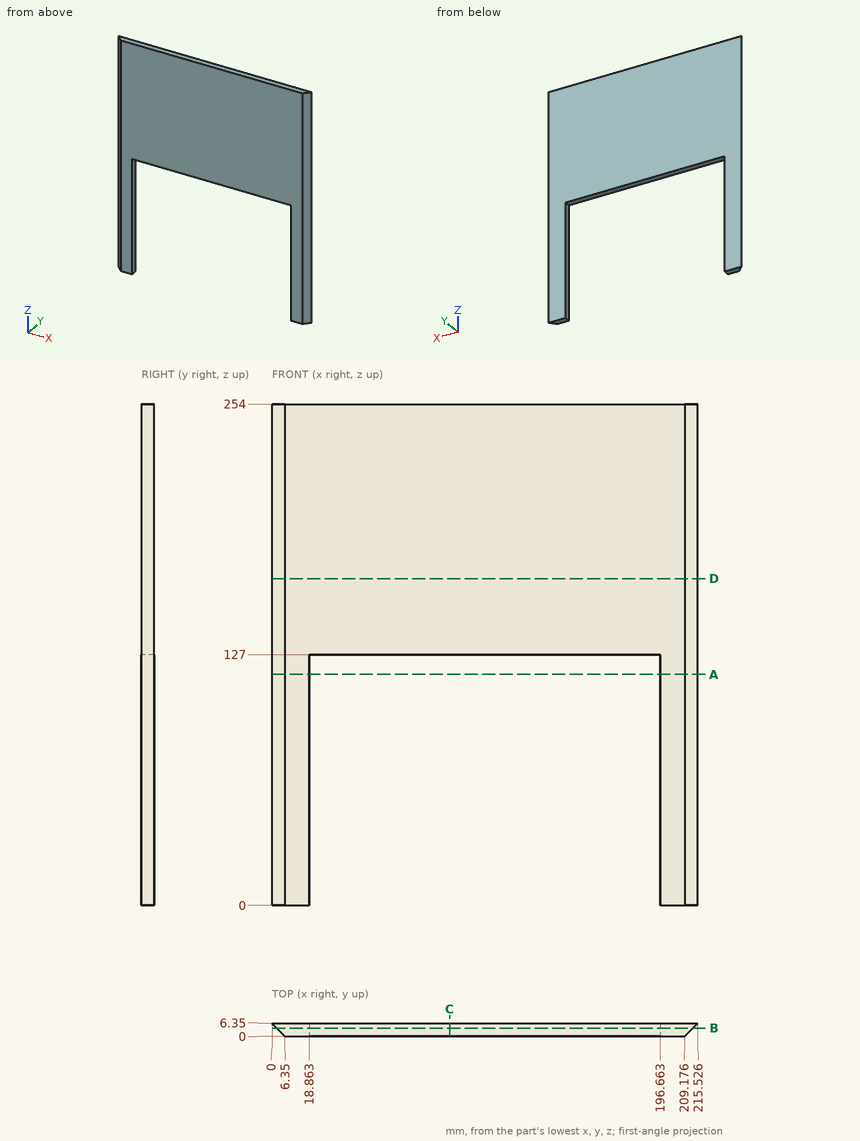
Input: dimensioned drawing with shaded views. Units: mm. Origin: part minimum x, y, z. Coordinates: 2 decimals unless noted, no trailing zeros. Order: outer loops, then holes, each group sorted by start corner. A loop starts at its lowest first (then second) coordinate and runs counter-clockwise, first axis right, second up. Notation, with made-up numbers: M 39,17 L 80,17 A25 ccw 80,34 Z; hole C -6,-39 d7. An arc over 180 degrees is marked long. Write each question's results on one line, items separated by ' | '. Start each with the question number.
Item 1: Cut plane B-B (y = 4). Return loops of the section in (x, z).
Item 2: Cut plane A-A (z = 117). Return loops of the section in (x, y), and give its area (3 significant figures).
Item 3: Cut plane D-D (z = 165.5). Return loops of the section in (x, y), and give its area (3 significant figures).
Item 4: First-contact query: pin 1 Ø3 at (y, z) = (3, 51.5) entering from +X; pin 2 Ø1.5 at (x, y) = (74, 2.5) entering from -Z; pin 3 Ø1 at (y, z) = (5, 147) entering from -X. Flat tips, straight axial feed; report the tip coordinate or a pass-through.
Item 5: Line query: probe 1 along Z at (x, y) = (109.5, 2.25); probe 2 along X at (y, z) = (5.5, 52.5); probe 3 along X at (y, z) = (4.5, 92). Output: solid intervals per line, ascending.
Item 6: Cut plane C-C (x = 90). Return loops of the section in (y, z).
Checked values:
1) outline: M 2.35,0 L 18.86,0 L 18.86,127 L 196.66,127 L 196.66,0 L 213.18,0 L 213.18,254 L 2.35,254 Z
2) outline: M 0,6.35 L 6.35,0 L 18.86,0 L 18.86,6.35 Z; M 196.66,0 L 209.18,0 L 215.53,6.35 L 196.66,6.35 Z | area: 199 mm2
3) outline: M 0,6.35 L 6.35,0 L 209.18,0 L 215.53,6.35 Z | area: 1,330 mm2
4) pin 1: stops at x = 213.68 | pin 2: stops at z = 127 | pin 3: stops at x = 0.85
5) probe 1: z = 127 to 254 | probe 2: x = 0.85 to 18.86, 196.66 to 214.68 | probe 3: x = 1.85 to 18.86, 196.66 to 213.68
6) outline: M 0,127 L 6.35,127 L 6.35,254 L 0,254 Z
